```python
from build123d import *

# Parameters (mm, degrees)
F1_DEPTH    = 25.4
F2_T1_DEPTH = 355.0052962601
F3_T1_DEPTH = 79.5444841249
F3_T3_DEPTH = 58.9324911013
F3_T6_ANGLE = 57.8558117321


# Not quite as in the source:
# - a fillet or chamfer that OpenCascade refuses, or shapes differently, is made with other operations: its cross-section is extruded or revolved along the edge and cut away or added


with BuildPart() as f1:
    # F0 (on Front) → F1 (new body)
    with BuildSketch(Plane.XZ):
        Polygon((16.8645065278, 28.9830360562), (0, 0), (62.5720471144, -6.3669001684), (62.5720471144, 25.0710807741), align=None)
    extrude(amount=F1_DEPTH)

    # F2: fillet of radius 76.2 on 1 edges, made by hand

    # F2_s2 → F2_t1 (cut)
    with BuildSketch(Plane.XZ.offset(-164.8026481301)):
        with BuildLine():
            ThreePointArc((62.5720471144, -40.849978478), (50.1292639894, 0.8807930983), (16.8645065278, 28.9830360562))
            Line((16.8645065278, 28.9830360562), (62.5720471144, 25.0710807741))
            Line((62.5720471144, 25.0710807741), (62.5720471144, -40.849978478))
        make_face()
    extrude(amount=F2_T1_DEPTH, mode=Mode.SUBTRACT)

    # F3: fillet of radius 5.08 on 3 edges, made by hand

    # F3_s2 → F3_t1 (cut)
    with BuildSketch(Plane(origin=(-12.6347602087, 0, 1.2856261), x_dir=(0, 1, 0), z_dir=(0.9948630086, 0, -0.1012304016))):
        with BuildLine():
            ThreePointArc((-20.32, 0), (-23.9121024484, 1.4878975516), (-25.4, 5.08))
            Line((-25.4, 5.08), (-25.4, 0))
            Line((-25.4, 0), (-20.32, 0))
        make_face()
    extrude(amount=F3_T1_DEPTH, mode=Mode.SUBTRACT)

    # F3_s4 → F3_t3 (cut)
    with BuildSketch(Plane(origin=(23.2517216099, 0, 39.9599884335), x_dir=(0, 1, 0), z_dir=(-0.5029303214, 0, -0.8643269588))):
        with BuildLine():
            ThreePointArc((-20.32, 0), (-23.9121024484, 1.4878975516), (-25.4, 5.08))
            Line((-25.4, 5.08), (-25.4, 0))
            Line((-25.4, 0), (-20.32, 0))
        make_face()
    extrude(amount=F3_T3_DEPTH, mode=Mode.SUBTRACT)

    # F3_s5 → F3_t6 (revolve, cut)
    with BuildSketch(Plane(origin=(-3.2129562092, 0, 0.8033671188), x_dir=(0, 1, 0), z_dir=(-0.9701334009, 0, 0.2425720192))):
        with BuildLine():
            ThreePointArc((-20.32, -33.2643114045), (-23.9121024484, -31.776413853), (-25.4, -28.1843114045))
            Line((-25.4, -28.1843114045), (-25.4, -33.2643114045))
            Line((-25.4, -33.2643114045), (-20.32, -33.2643114045))
        make_face()
    revolve(axis=Axis((-13.6279528859, -25.4, -40.8499784781), (0, 1, 0)), revolution_arc=F3_T6_ANGLE, mode=Mode.SUBTRACT)


solid = f1.part
```
The model under review builds one solid part; all positions refer to its coordinate system, in mm. Give positions to 0.01 mm unless a question says otherwise; leave off trailing zeros. Loops run counter-clockwise (first coordinate to the right, second up) from the corner with the lowest first, then second, coordinate; pieces in that order, holes last. Notation, with made-up numbers: (-37, 70) -> (16, 70) arc R29 cw to (16, 95) -> close; hole circle Ø2 at (45.5, -40). An arc over 180 degrees is marked (long way). Use CSV: the item, a comma, the result in double quotes.
1. To check wall thickness, follow probe 1 along X at (y, z) = (-3.5, 2); probe 2 along X at (y, z) = (-15, 3); probe 3 along Z at (x, y) = (18, -10.5). State the ranges of each line that lie inside material, in increasing order. Write a range as from..to.
Result:
probe 1,"x = 1.16..49.38"
probe 2,"x = 1.75..48.69"
probe 3,"z = -1.83..28.48"
2. Consider section B-B, the plane y = -22.25. Write out the cut boundary in (x, z), then the cut area to 3 significant figures.
Result:
outline,"(0.63, 0.32) -> (53.2, -5.03) arc R75.82 ccw to (17.02, 28.5) -> close"
area,"921 mm²"
3. For P1, Ø8, axis at x = 40, y = -21, coming from the -Z side; P2, Ø8, axis at y = -16, z = 13, coming from the -X side; P3, Ø4, axis at y = -6.5, z = 6.5, coming from the +X side; P4, Ø2, axis at x = 10, z = 1, coming from the +Y side, all flat-tipped, find the tip position at first contact; note any pin that passes through.
Result:
P1,"stops at z = -4.47"
P2,"stops at x = 5.24"
P3,"stops at x = 47.61"
P4,"stops at y = 0"
4. Consider section A-A, the plane y = -5.25. Write out the cut boundary in (x, z).
Result:
outline,"(0, 0) -> (53.87, -5.48) arc R76.2 ccw to (16.86, 28.98) -> close"
